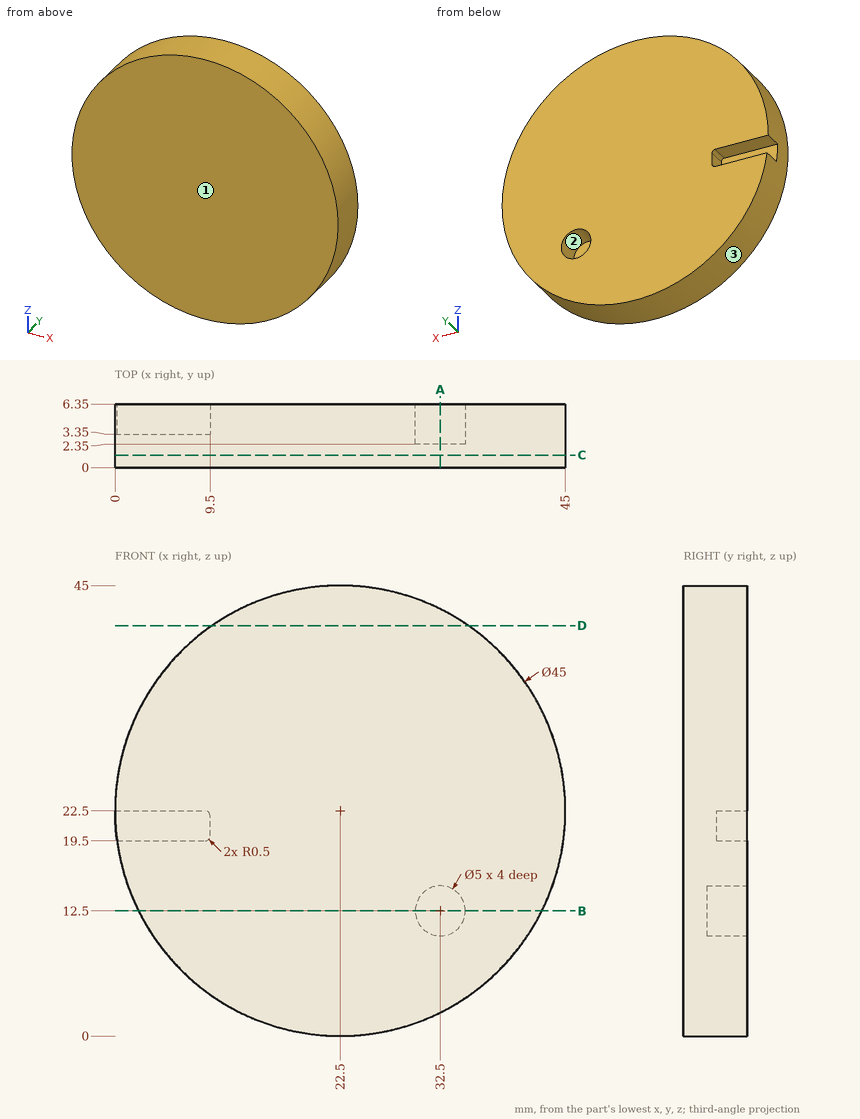
Geometry check sheet. Reference: drawing and pictorial views, mm from the part's lowest x, y, z. Round coordinates to 2 decimals unless told otherwise and drop trailing zeros. Loops run counter-clockwise (first coordinate to the right, second up) from the corner with the lowest first, then second, coordinate; pieces in that order, holes last. Notation, with made-up numbers: (5.5, 52) - (26.5, 52) arc R23 ccw to (26.5, 74) - close; hole circle Ø3 at (-28, 19.5). An arc over 180 degrees is marked (long way). One line per question, with ' | ' between items. Start each with the question number.
1. Cross-section at C-C on y = 1.25. Record the cut outline in (x, z).
2. Cross-section at A-A on x = 32.5. Record the cut outline in (y, z), then the cut area to 3 significant figures.
3. Depth check by flat-ended pin: pin 1 (1.5 mm diameter, centred on x = 33, z = 13.5, fed in from +Y); pin 2 (0.9 mm diameter, centred on x = 5.5, z = 20.5, fed in from +Y); pin 3 (1.6 mm diameter, centred on y = 5, z = 21, fed in from -X). Enter the tip coordinate at first touch or a pass-through.
4. Cross-section at D-D on z = 41. Record the cut outline in (x, y).
5. Cross-section at B-B on z = 12.5. Record the cut outline in (x, y).
6. Draft check along X on the marked faces 1, 2 and 3. Enter one of: released by +X, released by -X, zero draft, split by the parting line, or undercut.
7. Scan lines: line 1 (Z direction, x = 32.5, y = 3.3); line 2 (X direction, y = 3.75, z = 11); line 3 (X direction, y = 4.75, z = 23). Record each from-to range of solid material in increasing order. Write a range as [from, to].
Taken from the geometry:
1) outline: circle Ø45 at (22.5, 22.5)
2) outline: (0, 2.34) - (6.35, 2.34) - (6.35, 10) - (2.35, 10) - (2.35, 15) - (6.35, 15) - (6.35, 42.66) - (0, 42.66) - close | area: 236 mm²
3) pin 1: y = 2.35 | pin 2: y = 3.35 | pin 3: x = 9.5
4) outline: (9.69, 0) - (35.31, 0) - (35.31, 6.35) - (9.69, 6.35) - close
5) outline: (2.34, 0) - (42.66, 0) - (42.66, 6.35) - (35, 6.35) - (35, 2.35) - (30, 2.35) - (30, 6.35) - (2.34, 6.35) - close
6) face 1: zero draft | face 2: undercut | face 3: split by the parting line
7) line 1: [2.34, 10], [15, 42.66] | line 2: [3.16, 30.5], [34.5, 41.84] | line 3: [0.01, 44.99]
